Read the model definition and answer for the solid it produces. Units are mm, in the model's axes. A direction names the side the tool comes from. Give positions to 0.01 mm unless a question says otherwise; leave off trailing zeros. Order: outer loops, then holes, each group sorted by start corner. A loop starts at its lowest first (then second) coordinate and runs counter-clockwise, first axis right, second up. Notation, with made-up numbers: M 2,18 L 47,18 A10 cw 47,26 Z; hole C -17,71 d10. An arc over 180 degrees is marked long. One line per item, written item: value.
from build123d import *

# Parameters (mm, degrees)
F0_W      = 60
F0_H      = 40
F1_DEPTH  = 30
F3_DEPTH  = 20
F4_W      = 20
F4_H      = 10
F5_DEPTH  = 10
F6_W      = 40
F6_H      = 10
F7_DEPTH  = 25
F9_DEPTH  = 10
F11_DEPTH = 11
F13_DEPTH = 15
F16_DEPTH = 10
F18_DEPTH = 25


with BuildPart() as f1:
    # F0 (on Top) → F1 (new body)
    with BuildSketch(Plane.XY):
        with Locations((30, 20)):
            Rectangle(F0_W, F0_H)
    extrude(amount=F1_DEPTH)

    # F2 (on face) → F3 (cut)
    with BuildSketch(Plane.XY.offset(30)):
        Polygon((20, 10), (20, 0), (60, 0), (60, 30), (0, 30), (0, 10), align=None)
    extrude(amount=-F3_DEPTH, mode=Mode.SUBTRACT)

    # F4 (on face) → F5 (cut)
    with BuildSketch(Plane.XY.offset(30)):
        with Locations((10, 35)):
            Rectangle(F4_W, F4_H)
    extrude(amount=-F5_DEPTH, mode=Mode.SUBTRACT)

    # F6 (on face) → F7 (cut)
    with BuildSketch(Plane.XZ.offset(-30)):
        with Locations((40, 25)):
            Rectangle(F6_W, F6_H)
    extrude(amount=-F7_DEPTH, mode=Mode.SUBTRACT)

    # F10 (on face) → F11 (cut)
    with BuildSketch(Plane.XZ):
        with BuildLine():
            Line((20, 30), (10, 30))
            ThreePointArc((10, 30), (12.9289321881, 22.9289321881), (20, 20))
            Line((20, 20), (20, 30))
        make_face()
    extrude(amount=-F11_DEPTH, mode=Mode.SUBTRACT)


with BuildPart() as f9:
    # F8 (on face) → F9 (new body)
    with BuildSketch(Plane.XZ.offset(-30)):
        with BuildLine():
            Line((20.0364161283, 20), (60, 20))
            ThreePointArc((60, 20), (40.0182080641, 40.8581650258), (20.0364161283, 20))
        make_face()
    extrude(amount=-F9_DEPTH)


with BuildPart() as f13_tool:
    # F12 (on face) → F13 (new body)
    with BuildSketch(Plane.XZ.offset(-30)):
        with BuildLine():
            ThreePointArc((30, 20), (32.9289321881, 12.9289321881), (40, 10))
            ThreePointArc((40, 10), (47.0710678119, 12.9289321881), (50, 20))
            Line((50, 20), (40, 20))
            Line((40, 20), (30, 20))
        make_face()
        with BuildLine():
            Line((40, 20), (50, 20))
            ThreePointArc((50, 20), (40, 30), (30, 20))
            Line((30, 20), (40, 20))
        make_face()
    extrude(amount=-F13_DEPTH)


with BuildPart() as f1_1:
    add(f1.part)

    # F13: cut by f13_tool
    add(f13_tool.part, mode=Mode.SUBTRACT)

    # F15 (on face) → F16 (join)
    with BuildSketch(Plane.XZ.offset(-30)):
        with BuildLine():
            Line((50, 20), (60, 20))
            ThreePointArc((60, 20), (40, 40), (20, 20))
            Line((20, 20), (30, 20))
            Line((30, 20), (50, 20))
        make_face()
    extrude(amount=-F16_DEPTH)

    # F17 (on face) → F18 (cut)
    with BuildSketch(Plane.XZ.offset(-30)):
        with BuildLine():
            Line((30, 20), (50, 20))
            ThreePointArc((50, 20), (40, 30), (30, 20))
        make_face()
        with BuildLine():
            ThreePointArc((40, 10), (47.0710678119, 12.9289321881), (50, 20))
            Line((50, 20), (30, 20))
            ThreePointArc((30, 20), (32.9289321881, 12.9289321881), (40, 10))
        make_face()
    extrude(amount=-F18_DEPTH, mode=Mode.SUBTRACT)


with BuildPart() as f9_1:
    add(f9.part)

    # F13: cut by f13_tool
    add(f13_tool.part, mode=Mode.SUBTRACT)


solid = f1_1.part
1) Which of the six approach directions +Z, -Z, +X, -X, +Y, -Y give full straight-line access (tool end or side, diameter ignored) to faces 1 (the face through (30, 30, 22)), 2 (the face through (10, 35, 20)), 3 (the face through (20, 5, 15))?
Reported:
face 1: +Z, +X, -X
face 2: +Z, -X, +Y
face 3: +Z, +X, -Y
2) Consider probe 1 along Z at (x, y) = (39.5, 37); probe 2 along Z at (x, y) = (17.5, 32.5); probe 3 along Z at (x, y) = (12, 17.5). Determine where each line is inside the solid, lowest interval first.
Reported:
probe 1: z = 0 to 10.01, 29.99 to 39.99
probe 2: z = 0 to 20
probe 3: z = 0 to 10
3) Each of these flat-tipped pins is pushed along its axis until it touches: pin 1 Ø11 at (x, y) = (10.5, 34) entering from +Z; pin 2 Ø5 at (x, y) = (4, 6) entering from +Z; pin 3 Ø1.5 at (x, y) = (44.5, 22) entering from +Z. Where does it stop, or does it pass through?
Reported:
pin 1: stops at z = 20
pin 2: stops at z = 30
pin 3: stops at z = 10
4) Determine the mould class of faces 4 (the face through (23, 0, 8)), 5 (the face through (8, 10, 18)), 6 (the face through (0, 20, 8)) for opening direction Y: +Y half, -Y half, draft (parallel to the pull), parting line (faces both ways), or undercut.
Reported:
face 4: -Y half
face 5: undercut
face 6: draft
5) Find section B-B, the plane z = 16. Write down the section's boundary in (x, y), plus the area to 3 significant figures.
Reported:
outline: M 0,0 L 20,0 L 20,10 L 0,10 Z; M 0,30 L 30.83,30 L 30.83,40 L 0,40 Z; M 49.17,30 L 60,30 L 60,40 L 49.17,40 Z
area: 617 mm^2
6) Find section A-A, the plane x = 44.5. Write down the section's boundary in (y, z).
Reported:
outline: M 0,0 L 40,0 L 40,11.07 L 30,11.07 L 30,10 L 0,10 Z; M 30,28.93 L 40,28.93 L 40,39.49 L 30,39.49 Z
7) Find section C-C, the plane y = 26.5. Write down the section's boundary in (x, z), plus the area to 3 significant figures.
Reported:
outline: M 0,0 L 60,0 L 60,10 L 0,10 Z
area: 600 mm^2
8) Find section D-D, the plane x = 21.5. Write down the section's boundary in (y, z).
Reported:
outline: M 0,0 L 40,0 L 40,27.6 L 30,27.6 L 30,10 L 0,10 Z
